Geometry: final body of the model. Coordinates: model frame, mm. A direction names the side the tool comes from. Give positions to 0.01 mm unless a question says otherwise; leave off trailing zeros. Write each loop counter-clockwise with the first axis right and the second up, starting at its lowest first coordinate (ties: lowest second). Pieces come first, ordered by that corner, then holes. Notation, with made-up numbers: M 60.25,-39.5 L 106.25,-39.5 A8 ccw 106.25,-35.5 Z; hole C -21,2 d7. An arc over 180 degrees is marked long. Use a Markdown table: item, result. Add a question column.
(1) Draft query along Z for faces 5 (the flat face through (15751.034, -8420.644, -12931.885)), 6 (the flat face through (15751.85, -8421.07, -12926.62)), 7 (the cylindrical face through (15747.973, -8422.614, -12927.061)). Return one class per face: released by +Z, released by -Z, zero draft, split by the parting line, or undercut.
(2) Reachability of faces 1 (the flat face through (15750.776, -8415.915, -12927.919)), 2 (the flat face through (15745.591, -8417.756, -12924.284)), 3 (the flat face through (15751.4, -8420.8, -12930.3)), 4 (the cylindrical face through (15750.354, -8418.124, -12927.061)) from +Z, -Z, +X, -X, +Y, -Y: full face, straight path, thin tool, end or side. Return the list, or none.
(3) Cut plane B-B (y = -8415.5). Output: boundary loops of the cut face in (x, z).
(4) Material intervals for L1, parallel to Y at x = 15750.25, z = -12925.5; L2, parallel to X at y = -8420, z = -12925; L3, parallel to X at y = -8413.5, z = -12926.25, sorted ascending.
(5) Pin query (flat end, axial travel): pin 1 Ø6 at (x, z) = (15747.5, -12928) entering from +Y; pin 2 Ø1.5 at (y, z) = (-8418, -12928.5) entering from -X; pin 3 Ø3 at (x, y) = (15753.5, -8425.5) entering from -Z. Return the tip coordinate at first contact, or that it passes through.
(6) Cut plane A-A (x = 15753.5). Output: boundary loops of the cut face in (y, z).
Autodesk Inventor part; units mm, degrees
ref_plane "Work Plane1" through (-367703.1992, 632830.1242, 533306.3882) normal (-0.7430322, 0.6187428, -0.2550695) x (0.5860721, 0.7855909, 0.1984099)
ref_plane "YZ Plane" through (0, 0, 0) normal (1, 0, 0) x (0, 1, 0)
ref_plane "XZ Plane" through (0, 0, 0) normal (0, 1, 0) x (-1, 0, 0)
ref_plane "Work Plane1" through (-367703.1992, 632830.1242, 533306.3882) normal (-0.7430322, 0.6187428, -0.2550695) x (0.5860721, 0.7855909, 0.1984099)
sketch "Sketch1" plane through (15736.2978, -8215.3634, -12939.6422) normal (-0.8717195, 0.4624093, -0.1621198) x (0.4686085, 0.883406, 0)
  circle A0 centre (-111.4493, -109512.2066) radius 1.9
  circle A1 centre (-105.9197, -109447.9073) radius 1.9
  line L0 (-1, 8.962) -> (1, 8.962)
  arc A2 (-4.0236, -0.3508) -> (-14, 8.962) centre (-14, -1.038) ccw
  arc A3 (-4, -7.838) -> (-1, -10.838) centre (-1, -7.838) ccw
  line L1 (-1, -10.838) -> (1, -10.838)
  arc A4 (1, -10.838) -> (4, -7.838) centre (1, -7.838) ccw
  line L2 (-6.0031, -0.3508) -> (-3.9739, -0.3508)
  line L3 (-421.5485, 0.712) -> (525.8715, 0.712)
  arc A5 (-3.6711, -0.5438) -> (-3.9739, -0.3508) centre (-3.9739, -0.685) ccw
  line L4 (-3.2429, -1.398) -> (-3.6711, -0.5438)
  arc A6 (-3.2429, -1.398) -> (-2.8963, -1.6208) centre (-2.8963, -1.2398) ccw
  line L5 (-2.0007, -1.6208) -> (-2.8963, -1.6208)
  arc A7 (-2.0007, -1.6208) -> (-1.6554, -1.4008) centre (-2.0007, -1.2398) ccw
  line L6 (-1.2684, -0.5708) -> (-1.6554, -1.4008)
  arc A8 (-0.9231, -0.3508) -> (-1.2684, -0.5708) centre (-0.9231, -0.7318) ccw
  line L7 (-0.9231, -0.3508) -> (1.1061, -0.3508)
  arc A9 (1.4089, -0.5438) -> (1.1061, -0.3508) centre (1.1061, -0.685) ccw
  line L8 (1.8384, -1.4008) -> (1.4089, -0.5438)
  arc A10 (1.8384, -1.4008) -> (2.1837, -1.6208) centre (2.1837, -1.2398) ccw
  line L9 (3.0793, -1.6208) -> (2.1837, -1.6208)
  arc A11 (3.0793, -1.6208) -> (3.4234, -1.4033) centre (3.0793, -1.2398) ccw
  line L10 (3.8551, -0.4948) -> (3.4234, -1.4033)
  arc A12 (4.1569, -0.304) -> (3.8551, -0.4948) centre (4.1569, -0.6382) ccw
  line L11 (4.1569, -0.304) -> (6.1861, -0.304)
  arc A13 (-1, 8.962) -> (-4, 5.962) centre (-1, 5.962) ccw
  arc A14 (4, 5.962) -> (1, 8.962) centre (1, 5.962) ccw
  line L12 (-4, -0.6008) -> (-3.9739, -0.6008)
  arc A15 (-3.8967, -0.6516) -> (-3.9739, -0.6008) centre (-3.9739, -0.685) ccw
  line L13 (-3.8967, -0.6516) -> (-3.4682, -1.5065)
  arc A16 (-3.4682, -1.5065) -> (-2.8963, -1.8708) centre (-2.8963, -1.2398) ccw
  line L14 (-2.8963, -1.8708) -> (-2.0007, -1.8708)
  arc A17 (-2.0007, -1.8708) -> (-1.4289, -1.5065) centre (-2.0007, -1.2398) ccw
  line L15 (-1.4289, -1.5065) -> (-1.0418, -0.6765)
  arc A18 (-0.9231, -0.6008) -> (-1.0418, -0.6765) centre (-0.9231, -0.7318) ccw
  line L16 (-0.9231, -0.6008) -> (1.1061, -0.6008)
  arc A19 (1.1833, -0.6516) -> (1.1061, -0.6008) centre (1.1061, -0.685) ccw
  line L17 (1.1833, -0.6516) -> (1.6135, -1.5101)
  arc A20 (1.6135, -1.5101) -> (2.1837, -1.8708) centre (2.1837, -1.2398) ccw
  line L18 (2.1837, -1.8708) -> (3.0793, -1.8708)
  arc A21 (3.0793, -1.8708) -> (3.6492, -1.5106) centre (3.0793, -1.2398) ccw
  line L19 (3.6492, -1.5106) -> (4, -0.7723)
  arc A22 (4.1569, -0.554) -> (4.0809, -0.602) centre (4.1569, -0.6382) ccw
  line L20 (4.1569, -0.554) -> (6.1861, -0.554)
  line L21 (-4, -0.6008) -> (-4, -7.838)
  line L22 (-4, 5.962) -> (-4, 0.962)
  line L23 (-4, 0.712) -> (-4, -0.3508)
  line L24 (-421.5485, 0.962) -> (-4.202, 0.962)
  line L25 (4, 0.962) -> (4, 5.962)
  arc A23 (14, 8.962) -> (4.025, -0.3311) centre (14, -1.038) ccw
  arc A24 (4.0005, -0.9335) -> (4, -1.038) centre (14, -1.038) ccw
  line L26 (4, -7.838) -> (4, -0.7723)
  line L27 (4, -0.3431) -> (4, 0.712)
  line L28 (-4, 0.962) -> (4, 0.962)
  line L29 (4.202, 0.962) -> (525.8715, 0.962)
  point P0 (-116.6614, -15646.3059)
  dimension "d0" = 3
  dimension "d2" = 3
  dimension "d3" = 0.25
extrude "Extrusion1" add sketch "Sketch1" along normal blind 7 contours L0 A14 L25 L28 L22 A13 | L21 L12 A15 L13 A16 L14 A17 L15 A18 L16 A19 L17 A20 L18 A21 L19 L26 A24 A4 L1 A3
sketch "Sketch2" plane through (15730.1957, -8212.1265, -12940.777) normal (-0.8717195, 0.4624093, -0.1621198) x (0.4686085, 0.883406, 0)
  circle A0 centre (0, 4.962) radius 1.9
  line L0 (1, 8.962) -> (-1, 8.962)
  arc A1 (-1, 8.962) -> (-4, 5.962) centre (-1, 5.962) ccw
  line L1 (-4, 5.962) -> (-4, 0.962)
  line L2 (4, 0.962) -> (4, 5.962)
  arc A2 (4, 5.962) -> (1, 8.962) centre (1, 5.962) ccw
  circle A3 centre (0, -6.838) radius 1.9
  arc A4 (-4, -7.838) -> (-1, -10.838) centre (-1, -7.838) ccw
  line L3 (-1, -10.838) -> (1, -10.838)
  arc A5 (1, -10.838) -> (4, -7.838) centre (1, -7.838) ccw
  line L4 (4, -7.838) -> (4, -0.7723)
  line L5 (4, -0.7723) -> (4, 0.962)
  line L6 (-4, -7.838) -> (-4, 0.962)
  point P0 (-116.6614, -15646.3059)
extrude "Extrusion2" add sketch "Sketch2" along normal blind 1.5
move or copy body "Move Body1" bodies to move or copy 1 copy no rotation origin (0, 0, 0) rotation axis (-0.4686085, -0.883406, 0) rotation angle 90 translate (4249.9407, -2254.4088, -30671.5092)
move or copy body "Move Body2" bodies to move or copy 1 copy no translate (14.9738, 0, -3.187)
move or copy body "Move Body3" bodies to move or copy 1 copy no translate (0, -205.3427, 0)
move or copy body "Move Body4" bodies to move or copy 1 copy no translate (10, 0, 0)
move or copy body "Move Body5" bodies to move or copy 1 copy no translate (-10, 0, 0)
equation "\"d4\" = d3"
properties part number "belt-clamp"
Answer list:
| question | item | result |
|---|---|---|
| 1 | face 5 | released by -Z |
| 1 | face 6 | undercut |
| 1 | face 7 | released by +Z |
| 2 | face 1 | +Z, -Z, +X, +Y |
| 2 | face 2 | +Z, -X, +Y |
| 2 | face 3 | none |
| 2 | face 4 | +Z |
| 3 | outline | M 15740.99,-12925.13 L 15742.55,-12933.51 L 15749.99,-12932.43 L 15749.99,-12923.82 Z |
| 4 | L1 | -8424.69 to -8423.69, -8420.31 to -8418.33, -8417.57 to -8415.64 |
| 4 | L2 | 15741.48 to 15750.32, 15752.12 to 15758.4 |
| 4 | L3 | 15742.6 to 15746.22 |
| 5 | pin 1 | y = -8412.98 |
| 5 | pin 2 | x = 15740.66 |
| 5 | pin 3 | z = -12931.4 |
| 6 | outline | M -8426.42,-12931.08 L -8417.36,-12931.78 L -8417.36,-12930.26 L -8419.19,-12930.12 L -8417.36,-12924.91 L -8417.36,-12923.17 L -8426.42,-12922.47 Z |
